The listing builds one solid part. Answer for the finished solid, in the listing's coordinates (mm). Face numbers are marked on the shaded views. Give positions to 0.01 mm unless a question says otherwise; leave off trailing zeros. Write each loop counter-clockwise with the first axis right and the second up, starting at its lowest first coordinate (ties: lowest second). Pieces come first, ordered by that corner, then holes. Notation, with made-up numbers: (50, 82) -> (82, 82) arc R24 ccw to (82, 117) -> close; hole circle Ø1 at (-3.75, -33.5). An arc over 180 degrees is marked (long way). Use CSV: the item, a comma, the result in double quotes. Start each with the question number.
Autodesk Inventor part; units mm, degrees
ref_plane "YZ Plane" through (0, 0, 0) normal (1, 0, 0) x (0, 1, 0)
ref_plane "XZ Plane" through (0, 0, 0) normal (0, 1, 0) x (-1, 0, 0)
ref_plane "XY Plane" through (0, 0, 0) normal (0, 0, 1) x (1, 0, 0)
sketch "Sketch1" plane through (0, 0, 0) normal (0, 0, 1) x (1, 0, 0)
  line L0 (5, 0) -> (336, 0)
  line L1 (341, 5) -> (341, 96)
  line L2 (336, 101) -> (5, 101)
  line L3 (0, 96) -> (0, 5)
  arc A0 (5, 101) -> (0, 96) centre (5, 96) ccw
  arc A1 (0, 5) -> (5, 0) centre (5, 5) ccw
  arc A2 (341, 96) -> (336, 101) centre (336, 96) ccw
  arc A3 (336, 0) -> (341, 5) centre (336, 5) ccw
  line L4 (5, 101.2) -> (336, 101.2)
  arc A4 (341.2, 96) -> (336, 101.2) centre (336, 96) ccw
  line L5 (341.2, 96) -> (341.2, 5)
  arc A5 (336, -0.2) -> (341.2, 5) centre (336, 5) ccw
  line L6 (336, -0.2) -> (5, -0.2)
  arc A6 (-0.2, 5) -> (5, -0.2) centre (5, 5) ccw
  line L7 (-0.2, 5) -> (-0.2, 96)
  arc A7 (5, 101.2) -> (-0.2, 96) centre (5, 96) ccw
  line L8 (5, 104) -> (336, 104)
  arc A8 (344, 96) -> (336, 104) centre (336, 96) ccw
  line L9 (344, 96) -> (344, 5)
  arc A9 (336, -3) -> (344, 5) centre (336, 5) ccw
  line L10 (336, -3) -> (5, -3)
  arc A10 (-3, 5) -> (5, -3) centre (5, 5) ccw
  line L11 (-3, 5) -> (-3, 96)
  arc A11 (5, 104) -> (-3, 96) centre (5, 96) ccw
  point P0 (0, 0)
  point P1 (341, 101)
  point P2 (0, 101)
  dimension "d0" = 341
  dimension "d1" = 101
  dimension "d2" = 5
  dimension "d3" = 0.2
  dimension "d4" = 3
extrude "Extrusion1" add sketch "Sketch1" along normal blind 2 contours A1 L3 A0 L2 A2 L1 A3 L0 | L4 A4 L5 A5 L6 A6 L7 A7 | L8 A8 L9 A9 L10 A10 L11 A11
sketch "Sketch2" plane through (0, 0, 2) normal (0, 0, 1) x (1, 0, 0)
  line L0 (5, 104) -> (336, 104)
  line L1 (344, 96) -> (344, 5)
  line L2 (336, -3) -> (5, -3)
  line L3 (-3, 5) -> (-3, 96)
  line L4 (344, 5) -> (344, 96)
  line L5 (5, -3) -> (336, -3)
  arc A0 (5, 104) -> (-3, 96) centre (5, 96) ccw
  arc A1 (-3, 5) -> (5, -3) centre (5, 5) ccw
  arc A2 (336, -3) -> (344, 5) centre (336, 5) ccw
  arc A3 (344, 96) -> (336, 104) centre (336, 96) ccw
  line L6 (336, 101.2) -> (5, 101.2)
  arc A4 (5, 101.2) -> (-0.2, 96) centre (5, 96) ccw
  line L7 (-0.2, 96) -> (-0.2, 5)
  arc A5 (-0.2, 5) -> (5, -0.2) centre (5, 5) ccw
  line L8 (5, -0.2) -> (336, -0.2)
  arc A6 (336, -0.2) -> (341.2, 5) centre (336, 5) ccw
  line L9 (341.2, 5) -> (341.2, 96)
  arc A7 (341.2, 96) -> (336, 101.2) centre (336, 96) ccw
  circle A8 centre (5, 96) radius 2.5
  line L10 (9, 92) -> (332, 92)
  line L11 (332, 92) -> (332, 9)
  line L12 (332, 9) -> (9, 9)
  line L13 (9, 9) -> (9, 92)
  line L14 (-0.2, 89.2) -> (8, 89.2)
  line L15 (8, 89.2) -> (8, 93)
  line L16 (8, 93) -> (11.8, 93)
  line L17 (11.8, 93) -> (11.8, 101.2)
  line L18 (9, 9) -> (332, 92)
  line L19 (170.5, 64.427) -> (170.5, 38.8649)
  line L20 (118.7328, 50.5) -> (212.1169, 50.5)
  circle A9 centre (336, 96) radius 2.5
  line L21 (341.2, 89.2) -> (333, 89.2)
  line L22 (333, 89.2) -> (333, 93)
  line L23 (333, 93) -> (329.2, 93)
  line L24 (329.2, 93) -> (329.2, 101.2)
  circle A10 centre (5, 5) radius 2.5
  line L25 (-0.2, 11.8) -> (8, 11.8)
  line L26 (8, 11.8) -> (8, 8)
  line L27 (8, 8) -> (11.8, 8)
  line L28 (11.8, 8) -> (11.8, -0.2)
  line L29 (329.2, 8) -> (329.2, -0.2)
  line L30 (333, 8) -> (329.2, 8)
  line L31 (333, 11.8) -> (333, 8)
  line L32 (341.2, 11.8) -> (333, 11.8)
  circle A11 centre (336, 5) radius 2.5
  point P0 (0, 0)
  dimension "d7" = 0
  dimension "d8" = 0
  dimension "d9" = 8
  dimension "d10" = 2.8
  dimension "d11" = 5
  dimension "d12" = 5.2
  dimension "d13" = 5.2
  dimension "d19" = 9.2
  dimension "d20" = 9.2
  dimension "d21" = 9.2
  dimension "d22" = 9.2
  dimension "d23" = 1
  dimension "d24" = 1
  dimension "d25" = 12
  dimension "d26" = 12
extrude "Extrusion2" add sketch "Sketch2" along normal blind 30 contours L0 A3 L1 A2 L2 A1 L3 A0 | A7 L9 L21 L22 L23 L24 L6 | L17 L16 L15 L14 L7 A4 L6 | L9 A6 L8 L29 L30 L31 L32 | L25 L26 L27 L28 L8 A5 L7
sketch "Sketch3" plane through (0, 0, 32) normal (0, 0, 1) x (1, 0, 0)
  line L0 (5, 104) -> (336, 104)
  line L1 (344, 96) -> (344, 5)
  line L2 (336, -3) -> (5, -3)
  line L3 (-3, 5) -> (-3, 96)
  arc A0 (5, 104) -> (-3, 96) centre (5, 96) ccw
  arc A1 (-3, 5) -> (5, -3) centre (5, 5) ccw
  arc A2 (336, -3) -> (344, 5) centre (336, 5) ccw
  arc A3 (344, 96) -> (336, 104) centre (336, 96) ccw
  line L4 (336, 101.2) -> (5, 101.2)
  arc A4 (5, 101.2) -> (-0.2, 96) centre (5, 96) ccw
  line L5 (-0.2, 96) -> (-0.2, 5)
  arc A5 (-0.2, 5) -> (5, -0.2) centre (5, 5) ccw
  line L6 (5, -0.2) -> (336, -0.2)
  arc A6 (336, -0.2) -> (341.2, 5) centre (336, 5) ccw
  line L7 (341.2, 5) -> (341.2, 96)
  arc A7 (341.2, 96) -> (336, 101.2) centre (336, 96) ccw
  point P0 (0, 0)
  dimension "d29" = 8
  dimension "d30" = 2.8
extrude "Extrusion3" add sketch "Sketch3" along normal blind 7
sketch "Sketch4" plane through (0, 0, 2) normal (0, 0, 1) x (1, 0, 0)
  line L0 (336, -0.2) -> (5, -0.2)
  line L1 (157.75, -0.2) -> (183.25, -0.2)
  line L2 (183.25, -0.2) -> (183.25, 48.2)
  line L3 (183.25, 48.2) -> (157.75, 48.2)
  line L4 (157.75, 48.2) -> (157.75, -0.2)
  line L5 (-0.2, 5) -> (-0.2, 96)
  circle A0 centre (160.25, 45.7) radius 2.3
  circle A1 centre (180.75, 45.7) radius 2.3
  circle A2 centre (160.25, 2.3) radius 2.3
  circle A3 centre (180.75, 2.3) radius 2.3
  point P0 (0, 0)
  dimension "d33" = 25.5
  dimension "d34" = 48.4
  dimension "d35" = 157.95
  dimension "d36" = 4.6
  dimension "d37" = 4.6
  dimension "d38" = 4.6
  dimension "d39" = 4.6
  dimension "d40" = 2.5
  dimension "d41" = 2.5
  dimension "d42" = 2.5
  dimension "d43" = 2.5
  dimension "d44" = 2.5
  dimension "d45" = 2.5
  dimension "d46" = 2.5
  dimension "d47" = 2.5
extrude "Extrusion4" add sketch "Sketch4" along normal blind 4 contours A0 | A1 | A2 | A3
sketch "Sketch5" plane through (160.25, 2.3, 6) normal (0, 0, 1) x (1, 0, 0)
  circle A0 centre (0, 43.4) radius 2.3
  circle A1 centre (0, 43.4) radius 1.5
  circle A2 centre (20.5, 43.4) radius 2.3
  circle A3 centre (20.5, 43.4) radius 1.5
  circle A4 centre (0, 0) radius 2.3
  circle A5 centre (0, 0) radius 1.5
  circle A6 centre (20.5, 0) radius 2.3
  circle A7 centre (20.5, 0) radius 1.5
  point P0 (-160.25, -2.3)
  dimension "d50" = 3
  dimension "d51" = 3
  dimension "d52" = 3
  dimension "d53" = 3
extrude "Extrusion5" add sketch "Sketch5" along normal blind 3 contours A1 | A3
chamfer "Chamfer1" distance 1 angle 45 2 edges at (158.75, 45.7, 9) (179.25, 45.7, 9)
sketch "Sketch6" plane through (5, -3, 0) normal (0, -1, 0) x (1, 0, 0)
  line L0 (161.3, 2.8) -> (169.7, 2.8)
  line L1 (169.7, 2.8) -> (169.7, 6.2)
  line L2 (169.7, 6.2) -> (161.3, 6.2)
  line L3 (161.3, 6.2) -> (161.3, 2.8)
  line L4 (6.8, 2) -> (324.2, 2)
  line L5 (0, 0) -> (0, 39)
  point P0 (-5, 0)
  dimension "d59" = 8.4
  dimension "d60" = 3.4
  dimension "d61" = 4.2
  dimension "d62" = 161.3
extrude "Extrusion6" cut sketch "Sketch6" against normal blind 3
sketch "Sketch7" plane through (0, 0, 2) normal (0, 0, 1) x (1, 0, 0)
  line L0 (99.8, 7.8) -> (107.8, 7.8)
  line L1 (107.8, 7.8) -> (107.8, 10.8)
  line L2 (107.8, 10.8) -> (99.8, 10.8)
  line L3 (99.8, 10.8) -> (99.8, 7.8)
  line L4 (336, -0.2) -> (5, -0.2)
  line L5 (-0.2, 5) -> (-0.2, 96)
  point P0 (0, 0)
  dimension "d65" = 8
  dimension "d66" = 3
  dimension "d67" = 8
  dimension "d68" = 100
extrude "Extrusion7" cut sketch "Sketch7" against normal blind 3
sketch "Sketch8" plane through (0, 0, 2) normal (0, 0, 1) x (1, 0, 0)
  line L0 (11.8, -0.2) -> (329.2, -0.2)
  line L1 (95.8, -0.2) -> (111.8, -0.2)
  line L2 (111.8, -0.2) -> (111.8, 5.95)
  line L3 (111.8, 5.95) -> (95.8, 5.95)
  line L4 (95.8, 5.95) -> (95.8, -0.2)
  line L5 (107.8, 7.8) -> (99.8, 7.8)
  line L6 (99.8, 7.8) -> (99.8, 10.8)
  point P0 (0, 0)
  dimension "d71" = 16
  dimension "d72" = 1.85
  dimension "d73" = 4
extrude "Extrusion8" add sketch "Sketch8" along normal blind 9
properties part number "Case Full"
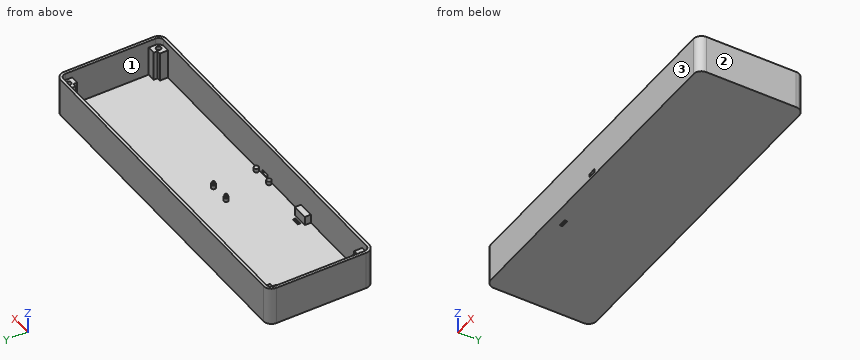
Q1. Section C-C on x = 209.5 is taken. Give the vertices of the cut face in (y, z).
Q2. Straight lines are drawn through the part: L1, parallel to Y at x = 5, z = 20; L2, parallel to X at y = 82, z = 18; L3, parallel to Y at x = 139.5, z = 28. For each, find the intervals that lie inside material, in ascending order.
Q3. The mould has two halves that part along X. Classify the marked faces 1, 2 and 3: +X half, -X half, draft (parallel to the pull), parting line (faces both ways), or undercut.
Q4. Flat-ended cylindrical pins translate along their axes: pin 1 Ø2.5 at (x, y) = (181.5, 2) entering from +Z; pin 2 Ø0.8 at (y, z) = (-2, 4.5) entering from +X; pin 3 Ø9 at (y, z) = (3, 22) entering from +X; pin 4 Ø4 at (x, y) = (101, 41) entering from +Z. Find the tip coordinate at first contact, or state that the pin passes through.
Q5. Section B-B on y = 16 is taken. Give the vertices of the cut face in (x, z), then the cut area to 3 significant figures.
Q6. Section A-A on z = 20 is taken. State how many separate pieces and enclosed holes the cut face has, then the cut area to 3 significant figures.
Output:
1,outline,"(-3, 0) -> (104, 0) -> (104, 39) -> (101.2, 39) -> (101.2, 2) -> (-0.2, 2) -> (-0.2, 39) -> (-3, 39) -> close"
2,L1,"-3 to 2.5, 7.5 to 11.8, 89.2 to 93.5, 98.5 to 104"
2,L2,"-3 to -0.2, 341.2 to 344"
2,L3,"-3 to -0.2, 101.2 to 104"
3,face 1,"undercut"
3,face 2,"+X half"
3,face 3,"draft"
4,pin 1,"z = 6"
4,pin 2,"x = 340.52"
4,pin 3,"x = 344"
4,pin 4,"z = 2"
5,outline,"(-3, 0) -> (344, 0) -> (344, 39) -> (341.2, 39) -> (341.2, 2) -> (-0.2, 2) -> (-0.2, 39) -> (-3, 39) -> close"
5,area,"901 mm²"
6,separate pieces,"1"
6,enclosed holes,"5"
6,area,"2,900 mm²"
